```python
from build123d import *

# Parameters (mm, degrees)
ESBO_O1_R                = 23.9
ESBO_O1_R_2              = 2
ESBO_O1_R_3              = 10
RESSALTO_EXTRUS_O1_DEPTH = 1.5
ESBO_O2_R                = 14
ESBO_O2_R_2              = 10
RESSALTO_EXTRUS_O2_DEPTH = 9.9
RESSALTO_EXTRUS_O3_START = -1.5
ESBO_O3_R                = 23.9
ESBO_O3_R_2              = 2
ESBO_O3_R_3              = 10
RESSALTO_EXTRUS_O3_DEPTH = 1.5
FILETE1_R                = 2


with BuildPart() as part:
    # Esboço1 → Ressalto-extrusão1 (new body)
    with BuildSketch(Plane.XY):
        Circle(ESBO_O1_R)
        with Locations((0, -20)):
            Circle(ESBO_O1_R_2, mode=Mode.SUBTRACT)
        with Locations((-17.320508076, -10)):
            Circle(ESBO_O1_R_2, mode=Mode.SUBTRACT)
        with Locations((-17.320508076, 10)):
            Circle(ESBO_O1_R_2, mode=Mode.SUBTRACT)
        with Locations((17.320508076, -10)):
            Circle(ESBO_O1_R_2, mode=Mode.SUBTRACT)
        with Locations((17.320508076, 10)):
            Circle(ESBO_O1_R_2, mode=Mode.SUBTRACT)
        with Locations((0, 20)):
            Circle(ESBO_O1_R_2, mode=Mode.SUBTRACT)
        Circle(ESBO_O1_R_3, mode=Mode.SUBTRACT)
    extrude(amount=RESSALTO_EXTRUS_O1_DEPTH)

    # Esboço2 → Ressalto-extrusão2 (add)
    with BuildSketch(Plane.XY.offset(1.5)):
        Circle(ESBO_O2_R)
        Circle(ESBO_O2_R_2, mode=Mode.SUBTRACT)
    extrude(amount=RESSALTO_EXTRUS_O2_DEPTH)

    # Esboço3 → Ressalto-extrusão3 (add)
    with BuildSketch(Plane.XY.offset(11.4).offset(RESSALTO_EXTRUS_O3_START)):
        Circle(ESBO_O3_R)
        with Locations((-17.320508076, -10)):
            Circle(ESBO_O3_R_2, mode=Mode.SUBTRACT)
        with Locations((0, -20)):
            Circle(ESBO_O3_R_2, mode=Mode.SUBTRACT)
        with Locations((17.320508076, -10)):
            Circle(ESBO_O3_R_2, mode=Mode.SUBTRACT)
        with Locations((17.320508076, 10)):
            Circle(ESBO_O3_R_2, mode=Mode.SUBTRACT)
        with Locations((0, 20)):
            Circle(ESBO_O3_R_2, mode=Mode.SUBTRACT)
        with Locations((-17.320508076, 10)):
            Circle(ESBO_O3_R_2, mode=Mode.SUBTRACT)
        Circle(ESBO_O3_R_3, mode=Mode.SUBTRACT)
    extrude(amount=RESSALTO_EXTRUS_O3_DEPTH)

    # Filete1
    filete1_edges = [part.edges().sort_by_distance(p)[0] for p in [
        (-14, 0, 1.5),
        (-14, 0, 9.9),
    ]]
    fillet(filete1_edges, radius=FILETE1_R)


solid = part.part
```
Geometry check sheet. Reference: the model listing, model coordinates, mm. A direction names the side the tool comes from. Round coordinates to 2 decimals unless told otherwise and drop trailing zeros. Loops run counter-clockwise (first coordinate to the right, second up) from the corner with the lowest first, then second, coordinate; pieces in that order, holes last. Notation, with made-up numbers: (88.25, -10.5) -> (125.25, -10.5) arc R19 ccw to (125.25, 13.5) -> close; hole circle Ø9 at (22, 79). An arc over 180 degrees is marked (long way). Use a Markdown table: item, result.
(1) Sectioned sample at D-D (x = 0). Give the number of separate pieces and of enclosed holes in the cut face, then the cut area to 3 significant figures.
Calculated:
| item | result |
|---|---|
| separate pieces | 6 |
| enclosed holes | 0 |
| area | 130 mm² |
(2) Set-up check for faces 5 (the flat face through (5, -16, 1.5)), 6 (the cylindrical face through (0, -18, 1)): record each of +Z, -Z, +X, -X, +Y, -Y from which the full face is reachable in a straight line by a thin tool's end or side.
Calculated:
| item | result |
|---|---|
| face 5 | none |
| face 6 | +Z, -Z |
(3) Sectioned sample at B-B (z = 10.75). Enter the section's corners in (x, y).
Calculated:
| item | result |
|---|---|
| outline | circle Ø47.8 at (0, 0); hole circle Ø4 at (-17.32, -10); hole circle Ø4 at (-17.32, 10); hole circle Ø20 at (0, 0); hole circle Ø4 at (0, -20); hole circle Ø4 at (0, 20); hole circle Ø4 at (17.32, -10); hole circle Ø4 at (17.32, 10) |
(4) Sectioned sample at C-C (x = 20). Enter the section's corners in (y, z), then the cut area to 3 significant figures.
Calculated:
| item | result |
|---|---|
| outline | (-13.08, 0) -> (13.08, 0) -> (13.08, 1.5) -> (-13.08, 1.5) -> close; (-13.08, 9.9) -> (13.08, 9.9) -> (13.08, 11.4) -> (-13.08, 11.4) -> close |
| area | 78.5 mm² |
(5) Mould release check, pull along Z, two halves, no side actions. Record for faces 1 (the cylindrical face through (0, -18, 11)), 2 (the cylindrical face through (12.932, -5.362, 5.669)), 3 (the flat face through (-0.3, -10.3, 11.4)), 4 (the flat face through (-0.3, -10.3, 0)): released by +Z, released by -Z, zero draft, split by the parting line, or undercut.
Calculated:
| item | result |
|---|---|
| face 1 | zero draft |
| face 2 | undercut |
| face 3 | released by +Z |
| face 4 | released by -Z |
(6) Sectioned sample at A-A (y = 0). Enter the section's corners in (x, z).
Calculated:
| item | result |
|---|---|
| outline | (-23.9, 0) -> (-10, 0) -> (-10, 11.4) -> (-23.9, 11.4) -> (-23.9, 9.9) -> (-16, 9.9) arc R2 cw to (-14, 7.9) -> (-14, 3.5) arc R2 cw to (-16, 1.5) -> (-23.9, 1.5) -> close; (10, 0) -> (23.9, 0) -> (23.9, 1.5) -> (16, 1.5) arc R2 cw to (14, 3.5) -> (14, 7.9) arc R2 cw to (16, 9.9) -> (23.9, 9.9) -> (23.9, 11.4) -> (10, 11.4) -> close |
(7) Scan lines: probe 1 along Y at (x, z) = (0, 11.05); probe 2 along Z at (x, y) = (3, 18); probe 3 along Y at (x, z) = (8, 10.5). Record each from-to range of solid material in increasing order.
Calculated:
| item | result |
|---|---|
| probe 1 | -23.9 to -22, -18 to -10, 10 to 18, 22 to 23.9 |
| probe 2 | 0 to 1.5, 9.9 to 11.4 |
| probe 3 | -22.52 to -6, 6 to 22.52 |
(8) Go/stop test with flat-tipped pins: P1, Ø3, axis at x = -17.32, y = 10, coming from the +Z side; P2, Ø1, axis at y = 12.5, z = 10, coming from the +X side; P3, Ø4, axis at x = -4, z = 8, coming from the +Y side; P4, Ø4, axis at y = 11, z = 6, coming from the -X side. Record where each tip stops, or that it passes through.
Calculated:
| item | result |
|---|---|
| P1 | through |
| P2 | x = 20.67 |
| P3 | y = 23.66 |
| P4 | x = -10.72 |
